Source: CAD feature listing. Evaluate the final solid. Frame: model axes, mm. A direction names the side the tool comes from. Round coordinates to 2 decimals unless told otherwise and drop trailing zeros. Loops run counter-clockwise (first coordinate to the right, second up) from the corner with the lowest first, then second, coordinate; pieces in that order, holes last.
(1) Section A-A, the plane z = 42. Return the cut outline in (x, y).
(2) Material intervals for probe 1 along Z at (x, y) = (-7.5, 10.25); probe 2 along Z at (x, y) = (6.5, -0.75); probe 3 along Y at (x, z) = (0, 4.5), sorted ascending.
(3) Section B-B, the plane z = 83. Return the cut outline in (x, y), plus the area to 3 significant figures.
(4) First-contact query: pin 1 Ø1.8 at (x, y) = (10, 0) entering from -Z; pin 2 Ø2 at (y, z) = (4.5, 70.5) entering from +X; pin 3 Ø1.5 at (x, z) = (3.5, 12) entering from -Y; pin 4 Ø8 at (y, z) = (-8.5, 68) entering from +X. Flat tips, straight axial feed; report the tip coordinate or a pass-through.
(5) Section C-C, the plane z = 31. Return the cut outline in (x, y), plus the area to 3 significant figures.
(6) Mould query, pull axis X, two halves, no side actions, for faces 4 (the cylindrical face through (0, 5, 60)), 5 (the flat face through (-6.4, 3.3, 5)), 6 (the cylindrical face through (0.75, -5.7, 91.92)). Classes: pulls with the +X half, pulls with the -X half, needs draft (parallel to the pull), parting line crosses it, or undercut.
(7) Set-up query: faces 1 (the flat face through (0, 3.5, 45)), 2 (the cylindrical face through (0.325, -11.464, 2.465)), 3 (the cylindrical face through (-1.301, -5.857, 48.078)). Return all of +Z, -Z, +X, -X, +Y, -Y with unobstructed straight access to the full face (end or side cutting, diameter ignored); none if empty.
```python
from build123d import *

# Parameters (mm, degrees)
SKETCH1_R                 = 15
BOSS_EXTRUDE1_DEPTH       = 5
SKETCH4_R                 = 1.5
CUT_EXTRUDE2_DEPTH        = 1
CUT_EXTRUDE2_DEPTH_BACK   = 6
SKETCH6_R                 = 6
BOSS_EXTRUDE2_DEPTH       = 90
CHAMFER1_SIZE             = 1
CUT_EXTRUDE3_DEPTH        = 2.5
SKETCH8_W                 = 0.25
SKETCH8_H                 = 1.15
F_5_0MM_DOWEL_HOLE1_D     = 5
F_5_0MM_DOWEL_HOLE1_DEPTH = 7.5
F_5_0MM_DOWEL_HOLE1_TIP   = 1.502151548
CHAMFER2_SIZE             = 1


with BuildPart() as part:
    # Sketch1 → Boss-Extrude1 (new body)
    with BuildSketch(Plane.XY):
        Circle(SKETCH1_R)
    extrude(amount=BOSS_EXTRUDE1_DEPTH)

    # Sketch4 → Cut-Extrude2 (cut, two sides)
    with BuildSketch(Plane(origin=(0, 0, 0), x_dir=(-1, 0, 0), z_dir=(0, 0, -1))) as cut_extrude2_sk:
        with Locations((10, 0)):
            Circle(SKETCH4_R)
        with Locations((0, -10)):
            Circle(SKETCH4_R)
        with Locations((-10, 0)):
            Circle(SKETCH4_R)
        with Locations((0, 10)):
            Circle(SKETCH4_R)
    extrude(amount=CUT_EXTRUDE2_DEPTH, mode=Mode.SUBTRACT)
    extrude(cut_extrude2_sk.sketch, amount=-CUT_EXTRUDE2_DEPTH_BACK, mode=Mode.SUBTRACT)

    # Sketch6 → Boss-Extrude2 (add)
    with BuildSketch(Plane.XY.offset(5)):
        Circle(SKETCH6_R)
    extrude(amount=BOSS_EXTRUDE2_DEPTH)

    # Chamfer1
    chamfer1_edges = [part.edges().sort_by_distance(p)[0] for p in [
        (-15, 0, 0),
        (-6, 0, 5),
        (-6, 0, 95),
        (-15, 0, 5),
    ]]
    chamfer(chamfer1_edges, length=CHAMFER1_SIZE)

    # Sketch7 → Cut-Extrude3 (cut)
    with BuildSketch(Plane(origin=(0, 6, 0), x_dir=(1, 0, 0), z_dir=(0, 1, 0))):
        with BuildLine():
            Line((-2.5, -57.5), (-2.5, -32.5))
            ThreePointArc((-2.5, -32.5), (0, -30), (2.5, -32.5))
            Line((2.5, -32.5), (2.5, -57.5))
            ThreePointArc((2.5, -57.5), (0, -60), (-2.5, -57.5))
        make_face()
    extrude(amount=-CUT_EXTRUDE3_DEPTH, mode=Mode.SUBTRACT)

    # Sketch8 → Cut-Revolve1 (revolve, cut)
    with BuildSketch(Plane(origin=(0, 0, 0), x_dir=(1, 0, 0), z_dir=(0, 1, 0))):
        with Locations((-5.875, -91.925)):
            Rectangle(SKETCH8_W, SKETCH8_H)
    revolve(axis=Axis((0, 0, 0), (0, 0, 1)), mode=Mode.SUBTRACT)

    # Ø5.0mm Dowel Hole1
    with Locations(Plane(origin=(0, 0, 0), x_dir=(-1, 0, 0), z_dir=(0, 0, -1))):
        with Locations((0, 0)):
            Hole(F_5_0MM_DOWEL_HOLE1_D / 2, depth=F_5_0MM_DOWEL_HOLE1_DEPTH)
            with Locations((0, 0, -(F_5_0MM_DOWEL_HOLE1_DEPTH + F_5_0MM_DOWEL_HOLE1_TIP / 2))):  # 118° drill point
                Cone(0, F_5_0MM_DOWEL_HOLE1_D / 2, F_5_0MM_DOWEL_HOLE1_TIP, mode=Mode.SUBTRACT)

    # Chamfer2
    chamfer2_edges = [part.edges().sort_by_distance(p)[0] for p in [
        (-2.5, 0, 0),
    ]]
    chamfer(chamfer2_edges, length=CHAMFER2_SIZE)


solid = part.part
```
Output values:
1. outline: (-2.5, 3.5) - (-2.5, 5.45) arc R6 ccw (long way) to (2.5, 5.45) - (2.5, 3.5) - close
2. probe 1: z = 0 to 5
2. probe 2: z = 0 to 5.46
2. probe 3: y = -14.5 to -11.5, -8.5 to -2.5, 2.5 to 8.5, 11.5 to 14.5
3. outline: circle Ø12 at (0, 0)
3. area: 113 mm2
4. pin 1: passes through
4. pin 2: stops at x = 4.87
4. pin 3: stops at y = -5.33
4. pin 4: stops at x = 3.97
5. outline: (-2, 3.5) - (-2, 5.66) arc R6 ccw (long way) to (2, 5.66) - (2, 3.5) - close
5. area: 104 mm2
6. face 4: undercut
6. face 5: needs draft
6. face 6: parting line crosses it
7. face 1: +Y
7. face 2: +Z, -Z
7. face 3: +Z
